Design review of the part built by this model. Coordinates are the model's own, in mm. Coordinates: 2 decimals unless noted, no trailing zeros. Write each loop counter-clockwise with the first axis right and the second up, starting at its lowest first coordinate (ties: lowest second). Pieces come first, ordered by that corner, then holes.
Q1. Add section A-A, the plane y = 7.25. Give the boundary of the cut face in (x, z).
Q2. Add section B-B, the plane x = 0. Give the boundary of the cut face in (y, z), plus the area to 3 significant figures.
Q3. The part is to be moulded in two halves that separate along X. For faces 1 (the face through (45, 10, -47)), 2 (the face through (2, 5, 69)), 3 (the face through (24.931, 4.93, 79.167)), say which applies: +X half, -X half, draft (parallel to the pull), parting line (faces both ways), or undercut.
Q4. Add section D-D, the plane z = -58.5. Give the boundary of the cut face in (x, y).
Q5. Add section C-C, the plane z = 0. Give the boundary of the cut face in (x, y), plus the area to 3 significant figures.
Q6. To check wall thickness, follow probe 1 along Z at (x, y) = (1, 3); probe 2 along Y at (x, z) = (61, -4); probe 3 along X at (y, z) = (6.75, -61). State the ranges of each line that lie inside material, in increasing order.
Q7. Clearance check with flat-ended pins moving along their axes: pin 1 Ø2 at (x, y) = (61.5, 7) entering from -Z; pin 2 Ø2 at (x, y) = (21, 9) entering from +Z; pin 3 Ø4 at (x, y) = (48.5, 7) entering from +Z. State where each tip first meets the part, or that it passes through.
from build123d import *

# Parameters (mm, degrees)
SKETCH1_R           = 83
BOSS_EXTRUDE1_DEPTH = 10
SKETCH3_R           = 56
CUT_EXTRUDE2_DEPTH  = 118.804923496
CUT_EXTRUDE4_START  = -5
CUT_EXTRUDE4_DEPTH  = 5


with BuildPart() as part:
    # Sketch1 → Boss-Extrude1 (new body)
    with BuildSketch(Plane(origin=(0, 0, 0), x_dir=(1, 0, 0), z_dir=(0, 1, 0))):
        with Locations(Location((0, 0, 0), (0, 0, 270))):
            Circle(SKETCH1_R)
    extrude(amount=BOSS_EXTRUDE1_DEPTH)

    # Sketch3 → Cut-Extrude2 (cut, through all)
    with BuildSketch(Plane.XZ):
        with Locations(Location((0, 0, 0), (0, 0, 270))):
            Circle(SKETCH3_R)
    extrude(amount=-CUT_EXTRUDE2_DEPTH, mode=Mode.SUBTRACT)

    # Sketch6 → Cut-Extrude4 (cut)
    with BuildSketch(Plane(origin=(0, 10, 0), x_dir=(1, 0, 0), z_dir=(0, 1, 0)).offset(CUT_EXTRUDE4_START)):
        with BuildLine():
            Line((55.715434798, -5.638290989), (79.539838583, -5.475879047))
            Line((79.539838583, -5.475879047), (82.819168969, -5.475879047))
            ThreePointArc((82.819168969, -5.475879047), (82.975116618, 2.032245607), (82.451795016, 9.523733443))
            Line((82.451795016, 9.523733443), (79.431867066, 9.523733443))
            Line((79.431867066, 9.523733443), (55.212462973, 9.358628767))
            ThreePointArc((55.212462973, 9.358628767), (55.968531574, 1.877091756), (55.715434798, -5.638290989))
        make_face()
        with BuildLine():
            Line((5.638290989, 55.715434798), (5.475879047, 79.539838583))
            Line((5.475879047, 79.539838583), (5.475879047, 82.819168969))
            ThreePointArc((5.475879047, 82.819168969), (-2.032245607, 82.975116618), (-9.523733443, 82.451795016))
            Line((-9.523733443, 82.451795016), (-9.523733443, 79.431867066))
            Line((-9.523733443, 79.431867066), (-9.358628767, 55.212462973))
            ThreePointArc((-9.358628767, 55.212462973), (-1.877091756, 55.968531574), (5.638290989, 55.715434798))
        make_face()
        with BuildLine():
            Line((-79.431867066, -9.523733443), (-55.212462973, -9.358628767))
            ThreePointArc((-55.212462973, -9.358628767), (-55.968531574, -1.877091756), (-55.715434798, 5.638290989))
            Line((-55.715434798, 5.638290989), (-79.539838583, 5.475879047))
            Line((-79.539838583, 5.475879047), (-82.819168969, 5.475879047))
            ThreePointArc((-82.819168969, 5.475879047), (-82.975116618, -2.032245607), (-82.451795016, -9.523733443))
            Line((-82.451795016, -9.523733443), (-79.431867066, -9.523733443))
        make_face()
        with BuildLine():
            Line((9.523733443, -79.431867066), (9.358628767, -55.212462973))
            ThreePointArc((9.358628767, -55.212462973), (1.877091756, -55.968531574), (-5.638290989, -55.715434798))
            Line((-5.638290989, -55.715434798), (-5.475879047, -79.539838583))
            Line((-5.475879047, -79.539838583), (-5.475879047, -82.819168969))
            ThreePointArc((-5.475879047, -82.819168969), (2.032245607, -82.975116618), (9.523733443, -82.451795016))
            Line((9.523733443, -82.451795016), (9.523733443, -79.431867066))
        make_face()
    extrude(amount=CUT_EXTRUDE4_DEPTH, mode=Mode.SUBTRACT)


solid = part.part
Here are the results:
1. outline: (-82.82, -5.48) arc R83 ccw to (-9.52, -82.45) - (-9.52, -79.43) - (-9.36, -55.21) arc R56 cw to (-55.72, -5.64) - (-79.54, -5.48) - close; (-82.45, 9.52) - (-79.43, 9.52) - (-55.21, 9.36) arc R56 cw to (-5.64, 55.72) - (-5.48, 79.54) - (-5.48, 82.82) arc R83 ccw to start; (5.48, -82.82) arc R83 ccw to (82.45, -9.52) - (79.43, -9.52) - (55.21, -9.36) arc R56 cw to (5.64, -55.72) - (5.48, -79.54) - close; (9.36, 55.21) arc R56 cw to (55.72, 5.64) - (79.54, 5.48) - (82.82, 5.48) arc R83 ccw to (9.52, 82.45) - (9.52, 79.43) - close
2. outline: (0, -83) - (5, -83) - (5, -56) - (0, -56) - close; (0, 56) - (5, 56) - (5, 83) - (0, 83) - close
2. area: 270 mm2
3. face 1: draft
3. face 2: undercut
3. face 3: parting line
4. outline: (-58.88, 0) - (58.88, 0) - (58.88, 10) - (5.62, 10) - (5.62, 5) - (-9.38, 5) - (-9.38, 10) - (-58.88, 10) - close
5. outline: (-83, 0) - (-56, 0) - (-56, 5) - (-83, 5) - close; (56, 0) - (83, 0) - (83, 5) - (56, 5) - close
5. area: 270 mm2
6. probe 1: z = -82.99 to -55.99, 55.99 to 82.99
6. probe 2: y = 0 to 5
6. probe 3: x = -56.28 to -9.4, 5.6 to 56.28
7. pin 1: stops at z = -56.82
7. pin 2: stops at z = 80.55
7. pin 3: stops at z = 68.75
